The model under review builds one solid part; all positions refer to its coordinate system, in mm. A direction names the side the tool comes from. Round coordinates to 2 decimals unless told otherwise and drop trailing zeros. Write each loop counter-clockwise with the first axis right and the second up, starting at its lowest first coordinate (ties: lowest second). Pieces come first, ordered by that corner, then holes. Notation, with made-up numbers: M -22,26.5 L -3,26.5 A9 ccw -3,33.5 Z; hole C -19,86 d8. An arc over 180 degrees is marked long. One line per item, written item: value. Start each with the question number.
1) Take a section at A-A, the plane y = -7. Write out the cut boundary in (x, z), and give its area (3 significant figures).
2) For P1, Ø1.2, axis at x = 10.5, z = -9.5, coming from the +Y side; P2, Ø1, axis at x = 1, z = 11.5, coming from the -Y side; P3, Ø1.5, axis at y = -4.5, z = -8, coming from the +X side, all flat-tipped, find the tip position at first contact; note any pin that passes through.
3) Tool access review of faces 1 (the face through (0, 15, 15)), 2 (the face through (11.91, 30.49, -13.52)), 3 (the face through (-7.5, 1, 0)), 4 (the face through (-12.209, 30.5, -9.8)), 5 (the face through (8.57, 30.49, -8.31)): name each direction out of +Z, -Z, +X, -X, +Y, -Y from which nothing blocks a thin tool from reaching the whole face with its end or side.
4) Wall thickness on probe 1 along Z at (x, y) = (2.25, 28); probe 2 along Z at (x, y) = (10.5, 30.6); probe 3 along Y at (x, z) = (-10, -12.9): over which ranges is each line inside the solid? List them lowest first.
5) Mouldability with a two-part tool opening along Z and no side actions: class faces 6 (the face through (9.75, 30.49, -9.8)), 7 (the face through (-11.924, 30.493, -13.504)), 8 (the face through (-5.3, -11.3, 11.5)), 9 (the face through (-1.446, 28.521, -10.017)) as +Z half, -Z half, draft (parallel to the pull), parting line (faces both ways), or undercut.
Autodesk Inventor part; units mm, degrees
ref_plane "Work Plane1" through (-11.0721, 29.5, 11.5458) normal (0, 0, 1) x (0, -1, 0)
ref_plane "YZ Plane" through (0, 0, 0) normal (1, 0, 0) x (0, 1, 0)
ref_plane "XZ Plane" through (0, 0, 0) normal (0, 1, 0) x (-1, 0, 0)
sketch "Sketch1" plane through (0, 0, 0) normal (0, 1, 0) x (-1, 0, 0)
  line L0 (-15, -15) -> (15, -15)
  line L1 (15, -15) -> (15, 15)
  line L2 (15, 15) -> (-15, 15)
  line L3 (-15, 15) -> (-15, -15)
  line L4 (-15, -15) -> (15, 15) construction
  line L5 (15, -15) -> (-15, 15) construction
  point P0 (0, 0)
  dimension "d0" = 30
  dimension "d1" = 30
extrude "Cube" add sketch "Sketch1" along normal blind 30
sketch "Sketch2" plane through (0, 0, 0) normal (0, -1, 0) x (1, 0, 0)
  circle A0 centre (0, 0) radius 14
  circle A1 centre (0, 0) radius 12.5
  dimension "d4" = 28
  dimension "d7" = 1.5
extrude "Lens Mount" add sketch "Sketch2" along normal blind 11.3
sketch "Sketch3" plane through (0, 0, 0) normal (0, -1, 0) x (1, 0, 0)
  line L0 (7.5, -5) -> (-7.5, -5)
  line L1 (-7.5, -5) -> (-7.5, 5)
  line L2 (-7.5, 5) -> (7.5, 5)
  line L3 (7.5, 5) -> (7.5, -5)
  line L4 (7.5, -5) -> (-7.5, 5) construction
  line L5 (-7.5, -5) -> (7.5, 5) construction
  point P0 (0, 0)
  dimension "d8" = 15
  dimension "d9" = 10
extrude "\"Sensor\"" cut sketch "Sketch3" against normal blind 2
sketch "Sketch4" plane through (15, 0, -15) normal (0, 0, -1) x (-1, 0, 0)
  line L0 (15, 0) -> (15, 30.669)
  line L1 (0, 30) -> (30, 30)
  point P0 (15, 26.85)
  point P1 (5, 3.15)
  point P2 (25, 3.15)
  dimension "d12" = 23.7
  dimension "d13" = 20
  dimension "d14" = 3.15
hole "Mounting Holes" at (0, 26.85, -15) at (10, 3.15, -15) at (-10, 3.15, -15) direction (0, 0, 1) diameter 3 depth 3 tip angle 118
sketch "Sketch5" plane through (0, 30, 0) normal (0, 1, 0) x (1, 0, 0)
  circle A0 centre (7.7053, -8.4968) radius 4
  circle A1 centre (7.7053, -8.4968) radius 3.2659
  point P0 (0, 0)
  dimension "d22" = 8
extrude "Cable Port" add sketch "Sketch5" along normal blind 5
sketch "Sketch6" plane through (0, 30, 0) normal (0, 1, 0) x (1, 0, 0)
  line L0 (7.2728, 8.793) -> (-7.0273, 8.793)
  line L1 (-7.0273, 8.793) -> (-6.3141, 10.6463)
  line L2 (-6.3141, 10.6463) -> (-2.7583, 10.6463)
  line L3 (-2.7583, 10.6463) -> (-2.3847, 9.4043)
  line L4 (-2.3847, 9.4043) -> (-1.5951, 9.4043)
  line L5 (-1.5951, 9.4043) -> (-1.2927, 10.6463)
  line L6 (-1.2927, 10.6463) -> (6.6007, 10.6463)
  line L7 (6.6007, 10.6463) -> (7.2728, 8.793)
  point P0 (0, 0)
extrude "HDMI profile" cut sketch "Sketch6" against normal blind 3
sketch "Sketch8" plane through (0, 30, 0) normal (0, 1, 0) x (1, 0, 0)
  line L0 (-7.5, 11.8014) -> (7.5, 11.8014)
  line L1 (9, 10.3014) -> (9, 9.362)
  line L2 (7.5, 7.862) -> (-7.5, 7.862)
  line L3 (-9, 9.362) -> (-9, 10.3014)
  line L4 (-9, 11.8014) -> (9, 7.862) construction
  line L5 (9, 11.8014) -> (-9, 7.862) construction
  arc A0 (7.5, 7.862) -> (9, 9.362) centre (7.5, 9.362) ccw
  arc A1 (-9, 9.362) -> (-7.5, 7.862) centre (-7.5, 9.362) ccw
  arc A2 (-7.5, 11.8014) -> (-9, 10.3014) centre (-7.5, 10.3014) ccw
  arc A3 (9, 10.3014) -> (7.5, 11.8014) centre (7.5, 10.3014) ccw
  line L6 (-11.209, 13.8051) -> (11.209, 13.8051)
  line L7 (12.209, 12.8051) -> (12.209, 6.8583)
  line L8 (11.209, 5.8583) -> (-11.209, 5.8583)
  line L9 (-12.209, 6.8583) -> (-12.209, 12.8051)
  line L10 (-12.209, 13.8051) -> (12.209, 5.8583) construction
  line L11 (12.209, 13.8051) -> (-12.209, 5.8583) construction
  arc A4 (11.209, 5.8583) -> (12.209, 6.8583) centre (11.209, 6.8583) ccw
  arc A5 (-12.209, 6.8583) -> (-11.209, 5.8583) centre (-11.209, 6.8583) ccw
  arc A6 (-11.209, 13.8051) -> (-12.209, 12.8051) centre (-11.209, 12.8051) ccw
  arc A7 (12.209, 12.8051) -> (11.209, 13.8051) centre (11.209, 12.8051) ccw
  circle A8 centre (10.5, 9.8317) radius 0.75
  circle A9 centre (-10.5, 9.8317) radius 0.75
  point P0 (0, 0)
  point P1 (0, 9.8317)
  dimension "d27" = 1.5
  dimension "d28" = 1
  dimension "d31" = 24.4179
  dimension "d32" = 18
  dimension "d33" = 1.5
  dimension "d34" = 10.5
  dimension "d35" = 1.5
  dimension "d36" = 10.5
extrude "Cable Mount" add sketch "Sketch8" along normal blind 1
sketch "Sketch9" plane through (0, 30, 0) normal (0, 1, 0) x (1, 0, 0)
  circle A0 centre (-11.0721, -11.5458) radius 1.5
  point P0 (0, 0)
  dimension "d37" = 3
extrude "Extrusion7" cut sketch "Sketch9" against normal blind 0.5
ref_plane "Work Plane1" through (-11.0721, 29.5, 11.5458) normal (0, 0, 1) x (0, -1, 0)
sketch "Sketch10" plane through (-11.0721, 29.5, 11.5458) normal (0, 0, 1) x (0, -1, 0)
  line L0 (0, -1.5) -> (0, 1.5)
  line L1 (0, -1.5) -> (0, 1.5)
  line L2 (-0.5, -1.5) -> (-0.5, 1.5)
  line L3 (0, -1.5) -> (0, 1.5)
  line L4 (-1.5, 0) -> (0, 0)
  arc A0 (-1.5, 0) -> (0, -1.5) centre (0, 0) ccw
  line L5 (-14.76, 0) -> (50.06, 0)
  point P0 (29.5, 11.0721)
  point P1 (0, 0)
revolve "Revolution1" add sketch "Sketch10" angle 360 about axis through (-11.0721, 29.5, 11.5458) along (0, -1, 0)
properties part number "OpticalCamera"
Checked values:
1. outline: C 0,0 d28; hole C 0,0 d25
1. area: 125 mm2
2. P1: stops at y = 31
2. P2: stops at y = 0
2. P3: stops at x = 11.98
3. face 1: +Z, +X, -X, +Y, -Y
3. face 2: -Z, +X, +Y
3. face 3: -Y
3. face 4: -Z, -X, +Y
3. face 5: +Y
4. probe 1: z = -15 to -10.65, -8.79 to 15
4. probe 2: z = -13.81 to -10.58, -9.08 to -5.86, 5.64 to 6.81, 10.19 to 11.36
4. probe 3: y = 0 to 1.65, 4.65 to 31
5. face 6: undercut
5. face 7: -Z half
5. face 8: draft
5. face 9: undercut
